Part model, mm, in its own coordinate system. A direction names the side the tool comes from. Coordinates: 2 decimals unless noted, no trailing zeros. Order: outer loops, then holes, each group sorted by start corner. A loop starts at its lowest first (then second) coordinate and runs counter-clockwise, first axis right, second up.
1) Cut at B-B (x = 16.25). List the corners of the cut face in (y, z), and give its area (3 significant figures).
2) Cut at A-A (y = 31.2). List the corners of the cut face in (x, z).
3) Cut at D-D (y = 4). List the corners of the cut face in (x, z).
4) Wall check: L1, parallel to Y at x = 24, z = 4.1; L2, parallel to X at y = 55.5, z = 1.45; L3, parallel to X at y = 44.5, z = 2.5. Give the ranges that are in metal, low to high.
5) Tool access for faces 1 (the flat face through (25.76, 41, 3)), 2 (the flat face through (0, 31, 3)), 3 (the flat face through (25.4, 3, 3)): list every direction of +Z, -Z, +X, -X, +Y, -Y with a clear straight run to the whole face (end or side of a thin tool).
6) Mould opens along Y. For faces 4 (the cylindrical face through (38.35, 43.74, 2.7)), 5 (the flat face through (32, 0, 3)), 6 (the flat face through (38.1, 3, 3)) say: +Y half, -Y half, draft (parallel to the pull), parting line (faces both ways), or undercut.
7) Cut at C-C (x = 39.5). List the corners of the cut face in (y, z).
8) Pin check, flat tips, straight feed: pin 1 Ø2.5 at (x, y) = (24, 44.62) entering from -Z; pin 2 Ø1.6 at (x, z) = (46, 3.5) entering from -Y. Stop position of each tip, or through.
```python
from build123d import *

# Parameters (mm, degrees)
SKETCH2_W           = 63.5
SKETCH2_H           = 63.5
BOSS_EXTRUDE1_DEPTH = 5.334
SKETCH4_W           = 12.7
SKETCH4_H           = 5.334
CUT_EXTRUDE1_DEPTH  = 5.334
SKETCH5_R           = 5.999999938
CUT_EXTRUDE2_DEPTH  = 5.334
SKETCH6_W           = 12
SKETCH6_H           = 44.450593975
CUT_EXTRUDE3_DEPTH  = 5.334
SKETCH7_R           = 1.45
CUT_EXTRUDE4_DEPTH  = 90.960833455


with BuildPart() as part:
    # Sketch2 → Boss-Extrude1 (new body)
    with BuildSketch(Plane.XY):
        with Locations((31.75, 31.75)):
            Rectangle(SKETCH2_W, SKETCH2_H)
    extrude(amount=BOSS_EXTRUDE1_DEPTH)

    # Sketch4 → Cut-Extrude1 (cut)
    with BuildSketch(Plane.XY.offset(5.334)):
        with Locations((19.05, 2.667)):
            Rectangle(SKETCH4_W, SKETCH4_H)
        with Locations((44.45, 2.667)):
            Rectangle(SKETCH4_W, SKETCH4_H)
    extrude(amount=-CUT_EXTRUDE1_DEPTH, mode=Mode.SUBTRACT)

    # Sketch5 → Cut-Extrude2 (cut)
    with BuildSketch(Plane.XY.offset(5.334)):
        with Locations((31.75, 18.699999938)):
            Circle(SKETCH5_R)
    extrude(amount=-CUT_EXTRUDE2_DEPTH, mode=Mode.SUBTRACT)

    # Sketch6 → Cut-Extrude3 (cut)
    with BuildSketch(Plane.XY.offset(5.334)):
        with Locations((31.76018242, 41.274703013)):
            Rectangle(SKETCH6_W, SKETCH6_H)
    extrude(amount=-CUT_EXTRUDE3_DEPTH, mode=Mode.SUBTRACT)

    # Sketch7 → Cut-Extrude4 (cut, through all)
    with BuildSketch(Plane.XY.offset(5.334)):
        with Locations((47.25, 31.199999957)):
            Circle(SKETCH7_R)
        with Locations((39.5, 17.776606198)):
            Circle(SKETCH7_R)
        with Locations((24, 17.776606198)):
            Circle(SKETCH7_R)
        with Locations((16.25, 31.199999957)):
            Circle(SKETCH7_R)
        with Locations((24, 44.623393716)):
            Circle(SKETCH7_R)
        with Locations((39.5, 44.623393716)):
            Circle(SKETCH7_R)
    extrude(amount=-CUT_EXTRUDE4_DEPTH, mode=Mode.SUBTRACT)


solid = part.part
```
Geometry check:
1. outline: (5.33, 0) - (29.75, 0) - (29.75, 5.33) - (5.33, 5.33) - close; (32.65, 0) - (63.5, 0) - (63.5, 5.33) - (32.65, 5.33) - close
1. area: 295 mm2
2. outline: (0, 0) - (14.8, 0) - (14.8, 5.33) - (0, 5.33) - close; (17.7, 0) - (25.76, 0) - (25.76, 5.33) - (17.7, 5.33) - close; (37.76, 0) - (45.8, 0) - (45.8, 5.33) - (37.76, 5.33) - close; (48.7, 0) - (63.5, 0) - (63.5, 5.33) - (48.7, 5.33) - close
3. outline: (0, 0) - (12.7, 0) - (12.7, 5.33) - (0, 5.33) - close; (25.4, 0) - (38.1, 0) - (38.1, 5.33) - (25.4, 5.33) - close; (50.8, 0) - (63.5, 0) - (63.5, 5.33) - (50.8, 5.33) - close
4. L1: y = 5.33 to 16.33, 19.23 to 43.17, 46.07 to 63.5
4. L2: x = 0 to 25.76, 37.76 to 63.5
4. L3: x = 0 to 22.56, 25.44 to 25.76, 37.76 to 38.06, 40.94 to 63.5
5. face 1: +Z, -Z, +Y
5. face 2: +Z, -Z, -X, +Y, -Y
5. face 3: +Z, -Z, -Y
6. face 4: undercut
6. face 5: -Y half
6. face 6: draft
7. outline: (5.33, 0) - (16.33, 0) - (16.33, 5.33) - (5.33, 5.33) - close; (19.23, 0) - (43.17, 0) - (43.17, 5.33) - (19.23, 5.33) - close; (46.07, 0) - (63.5, 0) - (63.5, 5.33) - (46.07, 5.33) - close
8. pin 1: passes through
8. pin 2: stops at y = 5.33
